from build123d import *

# Parameters (mm, degrees)
BOSS_EXTRUDE1_DEPTH = 1.6


with BuildPart() as part:
    # Sketch1 → Boss-Extrude1 (new body)
    with BuildSketch(Plane.ZY.offset(-5.18823967)):
        with BuildLine():
            ThreePointArc((10.414466289, -10.474403582), (10.727931837, -6.88180851), (7.135336765, -6.568342962))
            Line((7.135336765, -6.568342962), (-22.254454563, -31.241009834))
            ThreePointArc((-22.254454563, -31.241009834), (-22.567920111, -34.833604906), (-18.975325039, -35.147070454))
            Line((-18.975325039, -35.147070454), (10.414466289, -10.474403582))
        make_face()
        with BuildLine():
            ThreePointArc((10.324901527, -8.521373272), (10.179755112, -9.176267465), (9.771499716, -9.708509343))
            Line((9.771499716, -9.708509343), (-19.618291612, -34.381176215))
            ThreePointArc((-19.618291612, -34.381176215), (-21.802025871, -34.190638333), (-21.611487989, -32.006904073))
            Line((-21.611487989, -32.006904073), (7.778303338, -7.334237201))
            ThreePointArc((7.778303338, -7.334237201), (9.42979572, -7.116519687), (10.324901527, -8.521373272))
        make_face(mode=Mode.SUBTRACT)
    extrude(amount=BOSS_EXTRUDE1_DEPTH)


solid = part.part
Geometry check sheet. Reference: the model listing, model coordinates, mm. A direction names the side the tool comes from. Round coordinates to 2 decimals unless told otherwise and drop trailing zeros. Order: outer loops, then holes, each group sorted by start corner. A loop starts at its lowest first (then second) coordinate and runs counter-clockwise, first axis right, second up. Notation, with made-up numbers: M 54.5,33.5 L 65.5,33.5 A15 ccw 65.5,48.5 Z; hole C 17,26.5 d7. An arc over 180 degrees is marked long. Write each question's results on one line, items separated by ' | '. Start each with the question number.
1. Cross-section at C-C on y = -9.25. Record the boundary of the cut face in (x, z), plus the area to 3 significant figures.
2. Material ranges on L1, parallel to Z at x = 3.7, y = -10.5; L2, parallel to Z at x = 4.9, y = -24; L3, parallel to Y at x = 4.9, z = -16, recorded low to high. Write a range as from..to.
3. Set-up check for faces 1 (the face through (4.4, -19.84, -7.12)), 2 (the face through (3.588, -21, -9)): record each of +Z, -Z, +X, -X, +Y, -Y from which the full face is reachable in a straight line by a thin tool's end or side.
4. Cross-section at B-B on z = 6.5. Record the boundary of the cut face in (x, y).
5. Cross-section at A-A on x = 4.65. Record the boundary of the cut face in (y, z), plus the area to 3 significant figures.
6. Draft check along Y on faces 3 (the face through (4.399, -21.872, -4.718)), 4 (the face through (4.399, -6.925, 10.764)), 5 (the face through (4.4, -18.73, -7.35)). Enter one of: pulls with the +Y half, pulls with the -Y half, needs draft (parallel to the pull), parting line crosses it, or undercut.
Resolved:
1) outline: M 3.59,3.94 L 5.19,3.94 L 5.19,5.5 L 3.59,5.5 Z; M 3.59,10.14 L 5.19,10.14 L 5.19,11.22 L 3.59,11.22 Z | area: 4.21 mm2
2) L1: 2.45..4.01, 8.83..10.38 | L2: -13.63..-12.07, -7.25..-5.7 | L3: -32.65..-31.34, -27.3..-25.99
3) face 1: +X, -X | face 2: +Z, -Z, -X, +Y, -Y
4) outline: M 3.59,-13.76 L 5.19,-13.76 L 5.19,-12.45 L 3.59,-12.45 Z; M 3.59,-8.41 L 5.19,-8.41 L 5.19,-7.1 L 3.59,-7.1 Z
5) outline: M -35.15,-18.98 A2.55 ccw -31.24,-22.25 L -6.57,7.14 A2.55 ccw -10.47,10.41 Z; hole M -34.38,-19.62 A1.55 ccw -32.01,-21.61 L -7.33,7.78 A1.55 ccw -9.71,9.77 Z | area: 89.6 mm2
6) face 3: undercut | face 4: parting line crosses it | face 5: pulls with the +Y half
